Autodesk Inventor part; units mm, degrees
ref_plane "YZ Plane" through (0, 0, 0) normal (1, 0, 0) x (0, 1, 0)
ref_plane "XZ Plane" through (0, 0, 0) normal (0, 1, 0) x (-1, 0, 0)
ref_plane "XY Plane" through (0, 0, 0) normal (0, 0, 1) x (1, 0, 0)
sketch "Sketch1" plane through (0, 0, 0) normal (0, 1, 0) x (-1, 0, 0)
  circle A0 centre (0, 0) radius 53
  line L0 (-30.4755, 53.0714) -> (30.7235, 52.9283)
  line L1 (30.7235, 52.9283) -> (61.199, -0.1432)
  line L2 (61.199, -0.1432) -> (30.4755, -53.0714)
  line L3 (30.4755, -53.0714) -> (-30.7235, -52.9283)
  line L4 (-30.7235, -52.9283) -> (-61.199, 0.1432)
  line L5 (-61.199, 0.1432) -> (-30.4755, 53.0714)
  point P0 (-45.8372, 26.6073)
  dimension "d0" = 106
extrude "Extrusion1" add sketch "Sketch1" along normal blind 6
sketch "Sketch2" plane through (0, 6, 0) normal (0, 1, 0) x (1, 0, 0)
  circle A0 centre (0, 0) radius 19
  dimension "d3" = 38
extrude "Extrusion2" add sketch "Sketch2" along normal blind 4
sketch "Sketch3" plane through (0, 10, 0) normal (0, 1, 0) x (1, 0, 0)
  circle A0 centre (0, 0) radius 7
  dimension "d6" = 14
extrude "Extrusion3" cut sketch "Sketch3" against normal blind 10
fillet "Fillet1" radius 4 1 edges at (-19, 6, 0)
sketch "Sketch4" plane through (0, 0, 0) normal (0, -1, 0) x (1, 0, 0)
  circle A0 centre (0, 0) radius 45
  dimension "d10" = 90
extrude "Extrusion4" add sketch "Sketch4" along normal blind 5
sketch "Sketch5" plane through (0, -5, 0) normal (0, -1, 0) x (1, 0, 0)
  circle A0 centre (0, 0) radius 44
  dimension "d13" = 88
extrude "Extrusion5" add sketch "Sketch5" along normal blind 1
sketch "Sketch6" plane through (0, -6, 0) normal (0, -1, 0) x (1, 0, 0)
  circle A0 centre (0, 0) radius 40
  dimension "d16" = 80
extrude "Extrusion6" cut sketch "Sketch6" against normal blind 8
chamfer "Chamfer1" distance 1 angle 45 1 edges at (-44, -5, 0) measured on face at (33.706, -5.6667, -28.2827)
fillet "Fillet2" radius 2 7 edges at (-40, 2, 0) (-0.124, 0, 52.9999) (45.8372, 0, 26.6073) (-45.9612, 0, 26.3926) (-45.8372, 0, -26.6073) (45.9612, 0, -26.3926) (0.124, 0, -52.9999)
fillet "Fillet3" radius 5 12 edges at (30.3839, 0.5858, -52.3433) (30.7235, 4, -52.9283) (60.5226, 0.5858, 0.1416) (61.199, 4, 0.1432) (-30.4755, 4, -53.0714) (-30.1387, 0.5858, -52.4849) (30.4755, 4, 53.0714) (30.1387, 0.5858, 52.4849) (-30.7235, 4, 52.9283) (-30.3839, 0.5858, 52.3433) (-61.199, 4, -0.1432) (-60.5226, 0.5858, -0.1416)
sketch "Sketch9" plane through (0, 2, 0) normal (0, -1, 0) x (1, 0, 0)
  circle A0 centre (0, 0) radius 19
  dimension "d28" = 38
extrude "Extrusion7" add sketch "Sketch9" along normal blind 6
sketch "Sketch10" plane through (0, -4, 0) normal (0, -1, 0) x (1, 0, 0)
  circle A0 centre (0, 0) radius 14
  dimension "d31" = 28
extrude "Extrusion8" cut sketch "Sketch10" against normal blind 8
fillet "Fillet4" radius 2 1 edges at (-19, 2, 0)
sketch "Sketch11" plane through (0, 0, 0) normal (0, -1, 0) x (1, 0, 0)
  line L0 (0, 0) -> (-51, 0)
  circle A0 centre (-51, 0) radius 3.5
  dimension "d35" = 51
  dimension "d36" = 7
extrude "Extrusion9" cut sketch "Sketch11" against normal blind 10
pattern_circular "Circular Pattern1" count 6 over 360 about axis through (0, 10, 0) along (0, -1, 0) of "Extrusion9"
properties part number "crank case cover"
Check sheet for the modelled part. Datum: model origin and axes. Units: mm. A direction names the side the tool comes from. Coordinates: 2 decimals unless noted, no trailing zeros. Order: outer loops, then holes, each group sorted by start corner. A loop starts at its lowest first (then second) coordinate and runs counter-clockwise, first axis right, second up. Notation, with made-up numbers: (-12.5, -5) -> (11.5, -5) arc R18 cw to (11.5, 26) -> close; hole circle Ø11 at (-9, -22.75). An arc over 180 degrees is marked (long way). Write each question's results on one line, items separated by ' | '. Start each with the question number.
1) Section check A-A (y = -1.75). Enter the section's corners in (x, z), and give its area (3 significant figures).
2) Depth check by flat-ended pin: pin 1 (11 mm diameter, centred on x = 0, z = 0, fed in from -Y); pin 2 (5 mm diameter, centred on y = 6.5, z = 10.5, fed in from -X); pin 3 (14 mm diameter, centred on x = 1.5, z = 5.5, fed in from -Y); pin 4 (4 mm diameter, centred on x = -3, z = 26.5, fed in from +Y). Enter the tip coordinate at first touch or a pass-through.
3) Set-up check for faces 1 (the face through (1, 6, 24)), 2 (the face through (45.12, 0.57, 26.64)), 3 (the face through (-30, 0, -34)): record each of +Z, -Z, +X, -X, +Y, -Y from which the full face is reachable in a straight line by a thin tool's end or side.
4) Material ranges on line 1 along Z through (x, y) = (25.5, 2.35); line 2 along Z through (x, y) = (-25.5, 4); line 3 along X through (y, z) = (-0.75, 0.5), recorded low to high.
5) Draft check along X on faces 4 (the face through (12.932, -0.056, -5.362)), 5 (the face through (-46.032, 3.972, -26.272)), 6 (the face through (30.3, 3.97, -52.28)). Enter one of: pulls with the +X half, pulls with the -X half, needs draft (parallel to the pull), parting line crosses it, or undercut.
6) Section check B-B (z = 0). Count the separate pieces of the cut face and the enclosed holes in it, and give its area (3 significant figures).
Checked values:
1) outline: circle Ø90 at (0, 0); circle Ø38 at (0, 0); hole circle Ø80 at (0, 0); hole circle Ø28 at (0, 0) | area: 1,850 mm²
2) pin 1: through | pin 2: x = -56.49 | pin 3: y = 4 | pin 4: y = 6
3) face 1: +Y | face 2: +Z, +X, -Y | face 3: -Y
4) line 1: -52.94 to -47.67, -40.67 to 40.67, 47.67 to 53.06 | line 2: -53.06 to -47.67, -40.67 to 40.67, 47.67 to 52.94 | line 3: -45 to -40, -18.99 to -13.99, 13.99 to 18.99, 40 to 45
5) face 4: undercut | face 5: pulls with the -X half | face 6: pulls with the +X half
6) separate pieces: 4 | enclosed holes: 0 | area: 621 mm²
